Build history of the part. All positions in model axes, mm. A direction names the side the tool comes from. Round coordinates to 2 decimals unless told otherwise and drop trailing zeros. Loops run counter-clockwise (first coordinate to the right, second up) from the corner with the lowest first, then second, coordinate; pieces in that order, holes last. Notation, with made-up numbers: (-1, 52.5) - (9, 52.5) arc R5 ccw to (9, 58.5) - close; hole circle Ø1 at (48.5, -7). An arc over 180 degrees is marked (long way). Use a Markdown table: item, result.
from build123d import *

# Parameters (mm, degrees)
SKETCH011_W     = 20
SKETCH011_H     = 36
PAD004_DEPTH    = 25
SKETCH015_W     = 20
SKETCH015_H     = 10
PAD008_DEPTH    = 40
POCKET004_DEPTH = 10.001
SKETCH023_W     = 36
SKETCH023_H     = 88
SKETCH023_W_2   = 30
SKETCH023_H_2   = 85
PAD012_DEPTH    = 20
CHAMFER_SIZE    = 5
CHAMFER001_SIZE = 20
FILLET_R        = 3


with BuildPart() as part:
    # Sketch011 → Pad004 (new body)
    with BuildSketch(Plane(origin=(290, 240, 0), x_dir=(1, 0, 0), z_dir=(0, -1, 0))):
        with Locations((10, 15)):
            Rectangle(SKETCH011_W, SKETCH011_H)
    extrude(amount=-PAD004_DEPTH)

    # Sketch015 → Pad008 (join)
    with BuildSketch(Plane(origin=(0, 0, 33), x_dir=(-1, 0, 0), z_dir=(0, 0, 1))):
        with Locations((-300, -260)):
            Rectangle(SKETCH015_W, SKETCH015_H)
    extrude(amount=PAD008_DEPTH)

    # Sketch016 (on Face4 of Pad008) → Pocket004 (cut, through all)
    with BuildSketch(Plane.XZ.offset(-255)):
        with BuildLine():
            Line((299.941929, 43.5), (300.058071, 43.5))
            ThreePointArc((300.058071, 43.5), (303.022212, 44.727788), (304.25, 47.691929))
            Line((304.25, 47.691929), (304.25, 64.308071))
            ThreePointArc((304.25, 64.308071), (303.022212, 67.272212), (300.058071, 68.5))
            Line((300.058071, 68.5), (299.941929, 68.5))
            ThreePointArc((299.941929, 68.5), (296.977788, 67.272212), (295.75, 64.308071))
            Line((295.75, 64.308071), (295.75, 47.691929))
            ThreePointArc((295.75, 47.691929), (296.977788, 44.727788), (299.941929, 43.5))
        make_face()
    extrude(amount=-POCKET004_DEPTH, mode=Mode.SUBTRACT)

    # Sketch023 (on Face3 of Pocket004) → Pad012 (join)
    with BuildSketch(Plane(origin=(310, 0, 0), x_dir=(0, 0, 1), z_dir=(1, 0, 0))):
        with Locations((15, -196)):
            Rectangle(SKETCH023_W, SKETCH023_H)
        with Locations((16, -196.5)):
            Rectangle(SKETCH023_W_2, SKETCH023_H_2, mode=Mode.SUBTRACT)
    extrude(amount=-PAD012_DEPTH)

    # Chamfer
    chamfer_edges = [part.edges().sort_by_distance(p)[0] for p in [
        (300, 255, 33),
    ]]
    chamfer(chamfer_edges, length=CHAMFER_SIZE)

    # Chamfer001
    chamfer001_edges = [part.edges().sort_by_distance(p)[0] for p in [
        (300, 265, -3),
    ]]
    chamfer(chamfer001_edges, length=CHAMFER001_SIZE)

    # Fillet
    fillet_edges = [part.edges().sort_by_distance(p)[0] for p in [
        (300, 265, 73),
        (300, 255, 73),
        (300, 152, 33),
        (300, 152, -3),
        (300, 265, 17),
        (300, 245, -3),
    ]]
    fillet(fillet_edges, radius=FILLET_R)


with BuildPart() as part_1:
    # Body004 placement: moved
    add(part.part.moved(Location((0, 1, -1))))


solid = part_1.part
Q1. Which spindle directions (+Z, -Z, +X, -X, +Y, -Y) get a long thin tool onto all of the face, cutting with end or side? Do faces 1 (the face through (300, 204, 32)), 2 (the face through (300, 198, 30)), 3 (the face through (303.055, 260.93, 66.239)). Say none if no direction does.
Results found:
| item | result |
|---|---|
| face 1 | +Z, +X, -X, -Y |
| face 2 | +X, -X |
| face 3 | +Y, -Y |
Q2. Probe line 1 (Z direction, x = 308.5, y = 218.5); line 2 (X direction, y = 260.5, z = 52); line 3 (Y direction, x = 304.25, z = 44). List the from-to ranges inside material, lowest first.
Results found:
| item | result |
|---|---|
| line 1 | z = -4 to 0, 30 to 32 |
| line 2 | x = 290 to 295.75, 304.25 to 310 |
| line 3 | y = 256 to 266 |
Q3. Cut at A-A, the plane z = 2.5. List the corners of the cut face in (x, y).
Results found:
| item | result |
|---|---|
| outline | (290, 153) - (310, 153) - (310, 155) - (290, 155) - close; (290, 240) - (310, 240) - (310, 252.5) - (290, 252.5) - close |
Q4. Cut at C-C, the plane y = 227. List the corners of the cut face in (x, z).
Results found:
| item | result |
|---|---|
| outline | (290, -4) - (310, -4) - (310, 0) - (290, 0) - close; (290, 30) - (310, 30) - (310, 32) - (290, 32) - close |
Q5. Cut at D-D, the plane x = 302.5. List the corners of the cut face in (y, z).
Results found:
| item | result |
|---|---|
| outline | (153, -1) arc R3 ccw to (156, -4) - (244.76, -4) arc R3 ccw to (246.88, -3.12) - (265.12, 15.12) arc R3 ccw to (266, 17.24) - (266, 43.28) - (256, 43.28) - (256, 37) - (251, 32) - (156, 32) arc R3 ccw to (153, 29) - close; (256, 66.72) - (266, 66.72) - (266, 69) arc R3 ccw to (263, 72) - (259, 72) arc R3 ccw to (256, 69) - close; hole (155, 0) - (240, 0) - (240, 30) - (155, 30) - close |
Q6. Pull direction X, two halves, no side cores. Call faces 4 (the face through (300, 240, 15)), 5 (the face through (297.011, 260.93, 66.305)), 6 (the face through (290, 230, 31)): pulls with the +X half, pulls with the -X half, needs draft (parallel to the pull), parting line crosses it, or undercut.
Results found:
| item | result |
|---|---|
| face 4 | needs draft |
| face 5 | undercut |
| face 6 | pulls with the -X half |
Q7. Cut at B-B, the plane x = 308.5. List the corners of the cut face in (y, z).
Results found:
| item | result |
|---|---|
| outline | (153, -1) arc R3 ccw to (156, -4) - (244.76, -4) arc R3 ccw to (246.88, -3.12) - (265.12, 15.12) arc R3 ccw to (266, 17.24) - (266, 69) arc R3 ccw to (263, 72) - (259, 72) arc R3 ccw to (256, 69) - (256, 37) - (251, 32) - (156, 32) arc R3 ccw to (153, 29) - close; hole (155, 0) - (240, 0) - (240, 30) - (155, 30) - close |
Q8. Drop flat-ended pins along their axis: pin 1 (10 mm diameter, centred on x = 301, z = 9, fed in from +Y); pin 2 (12 mm diameter, centred on x = 305.5, z = 63, fed in from -Y); pin 3 (12 mm diameter, centred on x = 303, y = 253, fed in from -Z). Give the stop position or say it passes through.
Results found:
| item | result |
|---|---|
| pin 1 | stops at y = 264 |
| pin 2 | stops at y = 256 |
| pin 3 | stops at z = -3 |
